Autodesk Inventor part; units mm, degrees
ref_plane "Work Plane1" through (88.9, 0, 0) normal (1, 0, 0) x (0, 0, -1)
ref_plane "YZ Plane" through (0, 0, 0) normal (1, 0, 0) x (0, 1, 0)
ref_plane "XZ Plane" through (0, 0, 0) normal (0, 1, 0) x (-1, 0, 0)
sketch "Sketch1" plane through (0, 0, 0) normal (1, 0, 0) x (0, 1, 0)
  line L0 (0, 0) -> (95.25, 0)
  line L1 (0, 0) -> (0, -101.6)
  line L2 (0, -101.6) -> (6.35, -90.6015)
  line L3 (0, -101.6) -> (12.7, -101.6) construction
  arc A0 (66.6929, -89.0292) -> (95.25, -12.7) centre (71.7931, -47.4307) ccw
  arc A1 (57.0991, -96.1007) -> (95.25, 0) centre (66.6458, -44.2676) ccw
  arc A2 (57.0991, -96.1007) -> (66.6929, -89.0292) centre (51.9568, -79.0806) ccw
  arc A3 (95.25, -12.7) -> (6.35, -90.6015) centre (102.2308, -110.3428) ccw
  dimension "d18" = 101.6
  dimension "d20" = 12.7
  dimension "d21" = 60
  dimension "d27" = 41.91
  dimension "d28" = 52.705
  dimension "d29" = 17.78
  dimension "d30" = 57.099
  dimension "d31" = 66.6458
  dimension "d32" = 71.7931
  dimension "d33" = 95.25
  dimension "d34" = 66.6929
  dimension "d35" = 12.7
  dimension "d36" = 96.1007
  dimension "d38" = 74.276
extrude "Extrusion1" add sketch "Sketch1" along normal blind 177.8
sketch "Sketch2" plane through (177.8, 0, 0) normal (1, 0, 0) x (0, 0, -1)
  arc A0 (89.0292, 66.6929) -> (12.7, 95.25) centre (47.4307, 71.7931) ccw
  arc A1 (12.7, 95.25) -> (90.6015, 6.35) centre (110.3428, 102.2308) ccw
  line L0 (0, 95.25) -> (0, 0)
  arc A2 (96.1007, 57.0991) -> (89.0292, 66.6929) centre (79.0806, 51.9568) ccw
  line L1 (0, 58.8778) -> (0, 95.25)
  line L2 (0, 0) -> (101.6, 0)
  arc A3 (78.465, 69.7261) -> (36.7184, 37.715) centre (69.3573, 38.3767) ccw
  arc A4 (96.1007, 57.0991) -> (78.465, 69.7261) centre (47.1123, 7.3079) ccw
  line L3 (0, 58.8778) -> (36.7184, 37.715)
  arc A5 (96.1007, 57.0991) -> (0, 95.25) centre (44.2676, 66.6458) ccw
  arc A6 (96.1007, 57.0991) -> (0, 95.25) centre (44.2676, 66.6458) ccw
  arc A7 (12.7, 95.25) -> (36.7184, 37.715) centre (110.3428, 102.2308) ccw
  arc A8 (89.0292, 66.6929) -> (12.7, 95.25) centre (47.4307, 71.7931) ccw
  arc A9 (96.1007, 57.0991) -> (89.0292, 66.6929) centre (79.0806, 51.9568) ccw
  dimension "d49" = 21.1628
  dimension "d50" = 32.6457
  dimension "d51" = 69.85
  dimension "d52" = 16.8716
  dimension "d53" = 59.3379
ref_plane "Work Plane1" through (88.9, 0, 0) normal (1, 0, 0) x (0, 0, -1)
extrude "Extrusion2" add sketch "Sketch2" against normal blind 2.54
fillet "Fillet3" radius 19.05 1 edges at (176.53, 37.715, -36.7184)
mirror "Mirror1" about plane through (88.9, 0, 0) normal (1, 0, 0) of "Extrusion2", "Fillet3"
fillet "Fillet2" radius 19.05 2 edges at (88.9, 0, 0) (88.9, 95.25, 0)
sketch "Sketch3" plane through (2.54, 71.7931, -47.4307) normal (1, 0, 0) x (0, -0.3504094, -0.9365966)
  arc A0 (50.7331, 3.2921) -> (40.7482, 9.7997) centre (36.594, -7.4882) ccw
  arc A1 (40.7482, 9.7997) -> (-40.7482, 9.7997) centre (0, 0) ccw
  arc A2 (50.7331, 3.2921) -> (29.7909, 8.9388) centre (22.298, -60.5081) ccw
  arc A3 (50.7331, 3.2921) -> (-50.3771, 12.9226) centre (-1.1589, -5.9293) ccw
  arc A4 (50.7331, 3.2921) -> (40.7482, 9.7997) centre (36.594, -7.4882) ccw
  arc A5 (41.3731, 6.6868) -> (40.7482, 9.7997) centre (0, 0) ccw
  arc A6 (50.7331, 3.2921) -> (29.7909, 8.9388) centre (22.298, -60.5081) ccw
  arc A7 (-35.8187, -21.7593) -> (-43.5602, -37.2333) centre (22.298, -60.5081) ccw
  arc A8 (50.7331, 3.2921) -> (41.3731, 6.6868) centre (22.298, -60.5081) ccw
  point P0 (-19.2665, -83.8613)
extrude "Extrusion3" add sketch "Sketch3" along normal up to next
sketch "Sketch4" plane through (177.8, 0, 0) normal (1, 0, 0) x (0, 0, -1)
  arc A0 (96.1007, 57.0991) -> (4.7759, 101.5489) centre (44.2676, 66.6458) ccw
  line L0 (19.05, 0) -> (101.6, 0)
  arc A1 (96.1007, 57.0991) -> (4.7759, 101.5489) centre (44.2676, 66.6458) ccw
  point P0 (0, 0)
  point P1 (44.2676, 119.3508)
  dimension "d57" = 119.3508
properties part number "plowV2"
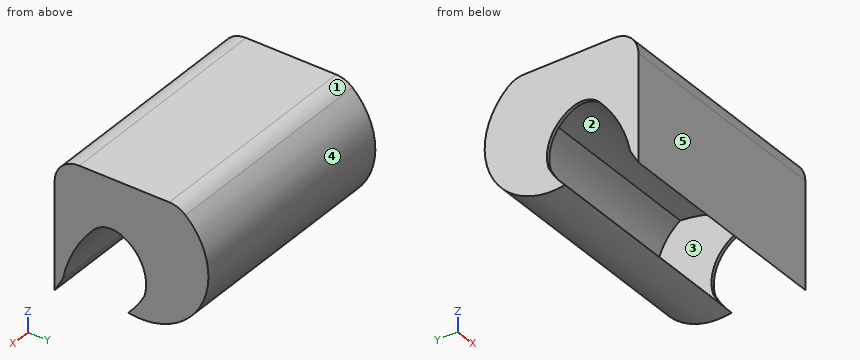
Source: CAD feature listing. Evaluate the final solid. Frame: model axes, mm. Face numbers are marked on the shaded views. A direction names the side the tool comes from. Give positions to 0.01 mm unless a question says otherwise; leave off trailing zeros. Order: outer loops, then holes, each group sorted by start corner. A loop starts at its lowest first (then second) coordinate and runs counter-clockwise, first axis right, second up. Notation, with made-up numbers: (27.5, -29.5) -> (36.5, -29.5) arc R6 ccw to (36.5, -22.5) -> close; hole circle Ø7 at (68, 39.5). An arc over 180 degrees is marked (long way). Use a Markdown table: item, result.
Q1. Pull-direction query (Z, two-part tool) for the marked faces 3, 4 and 5; classes: +Z half, -Z half, draft (parallel to the pull), parting line (faces both ways), or undercut.
A:
| item | result |
|---|---|
| face 3 | undercut |
| face 4 | parting line |
| face 5 | draft |
Q2. First-contact query: P1, Ø5, axis at x = 84.5, y = 45, coming from the -Z side; P2, Ø5, axis at x = 114, y = 79, coming from the -Z side; P3, Ø1.5, axis at x = 34, z = -33.5, coming from the +Y side. Flat tips, straight axial feed; report the tip coordinate or a pass-through.
A:
| item | result |
|---|---|
| P1 | z = -32.79 |
| P2 | z = -96.04 |
| P3 | y = 118.39 |
Q3. Section A-A (z = -85). Return the cut outline in (x, y), and give its area (3 significant figures).
A:
| item | result |
|---|---|
| outline | (0, 0) -> (177.8, 0) -> (177.8, 7.68) -> (0, 7.68) -> close; (0, 65.99) -> (2.54, 65.99) -> (2.54, 90.37) -> (175.26, 90.37) -> (175.26, 65.99) -> (177.8, 65.99) -> (177.8, 100.09) -> (0, 100.09) -> close |
| area | 3,220 mm^2 |
Q4. Section B-B (y = 77). Return the cut outline in (x, z).
A:
| item | result |
|---|---|
| outline | (0, -95.95) -> (177.8, -95.95) -> (177.8, 0) -> (0, 0) -> close; hole (2.54, -89.02) -> (175.26, -89.02) -> (175.26, -15.76) -> (2.54, -15.76) -> close |
Q5. Access query for the marked faces 1 and 2. Directions: +Z, -Z, +X, -X, +Y, -Y. A direction counts if a zero-diameter tool reaches every point of the face in a straight line with its end or side. Return the directions, or none.
A:
| item | result |
|---|---|
| face 1 | +Z, +X, -X, +Y |
| face 2 | none |
Q6. Material intervals for line 1 (X direction, y = 84.5, z = -38); line 2 (Y direction, x = 8.5, z = -64); line 3 (Z direction, x = 69, y = 94.5), sorted ascending. Write a range as [from, to].
A:
| item | result |
|---|---|
| line 1 | [0, 2.54], [175.26, 177.8] |
| line 2 | [0, 16], [110.29, 115.52] |
| line 3 | [-89.01, -82.66], [-12.76, -0.83] |
Q7. Section C-C (z = -31.5). Return the cut outline in (x, y).
A:
| item | result |
|---|---|
| outline | (0, 0) -> (177.8, 0) -> (177.8, 117.78) -> (0, 117.78) -> close; hole (2.54, 44.21) -> (175.26, 44.21) -> (175.26, 110.56) -> (2.54, 110.56) -> close |
